```python
from build123d import *

# Parameters (mm, degrees)
SKETCH1_R           = 35
BOSS_EXTRUDE1_DEPTH = 15
CHAMFER2_SIZE       = 7
SKETCH2_R           = 22.041880944
CUT_EXTRUDE1_DEPTH  = 7


with BuildPart() as part:
    # Sketch1 → Boss-Extrude1 (new body)
    with BuildSketch(Plane(origin=(0, 0, 0), x_dir=(1, 0, 0), z_dir=(0, 1, 0))):
        with Locations(Location((1.345738872, 0, 0), (0, 0, 270))):
            Circle(SKETCH1_R)
    extrude(amount=BOSS_EXTRUDE1_DEPTH)

    # Chamfer2
    chamfer2_edges = [part.edges().sort_by_distance(p)[0] for p in [
        (1.345738872, 0, -35),
    ]]
    chamfer(chamfer2_edges, length=CHAMFER2_SIZE)

    # Sketch2 → Cut-Extrude1 (cut)
    with BuildSketch(Plane(origin=(0, 15, 0), x_dir=(1, 0, 0), z_dir=(0, 1, 0))):
        with Locations(Location((0, 0, 0), (0, 0, 270))):
            Circle(SKETCH2_R)
    extrude(amount=-CUT_EXTRUDE1_DEPTH, mode=Mode.SUBTRACT)


solid = part.part
```
Work out the finished part from the listing and answer in its coordinate system (mm). A direction names the side the tool comes from. Coordinates: 2 decimals unless noted, no trailing zeros. Loops run counter-clockwise (first coordinate to the right, second up) from the corner with the lowest first, then second, coordinate; pieces in that order, holes last. Notation, with made-up numbers: M -32,1.5 L 1,1.5 A27 cw 1,33.5 Z; hole C 44,82.5 d10. An arc over 180 degrees is marked long. Use CSV: the item, a comma, the result in double quotes. Start each with the question number.
(1) Find section A-A, the plane z = 0. Give the vertices of the cut face in (x, y).
(2) For faces 4 (the face through (17, 15, 15)), 5 (the face through (6.621, 11.549, 21.024)), determine the directions among +Z, -Z, +X, -X, +Y, -Y from which every point of the face is accessible in a straight line to the end or side of a thin tool.
(3) For a pull along X with two mould halves and no side action, classify faces 1 (the face through (36.048, 10.944, -4.556)), 2 (the face through (2, 0, 0)), 3 (the face through (0, 8, 0)) as +X half, -X half, draft (parallel to the pull), parting line (faces both ways), or undercut.
(4) Find section C-C, the plane y = 4.75. Give the vertices of the cut face in (x, z), then the cut area to 3 significant figures.
(5) Find section B-B, the plane y = 11. Give the vertices of the cut face in (x, z), then the cut area to 3 significant figures.
(6) Given pin 1 Ø4 at (x, y) = (-10, 4.5) entering from -Z; pin 2 Ø10 at (x, z) = (4.5, 0) entering from +Y; pin 3 Ø8 at (x, y) = (15, 11) entering from +Z, each flat-ended and moving along its own axis, determine where each tip first touches the part or whether it passes through.
(7) Consider line 1 (X direction, y = 13.25, z = 0); line 2 (X direction, y = 9.5, z = 4.5); line 3 (Y direction, x = -6, z = -19.5). Determine where each line is inside the solid, lowest interval first.
Recorded:
1,outline,"M -33.65,7 L -26.65,0 L 29.35,0 L 36.35,7 L 36.35,15 L 22.04,15 L 22.04,8 L -22.04,8 L -22.04,15 L -33.65,15 Z"
2,face 4,"+Z, -Z, +X, -X, +Y"
2,face 5,"+Y"
3,face 1,"parting line"
3,face 2,"draft"
3,face 3,"undercut"
4,outline,"C 1.35,0 d65.5"
4,area,"3,370 mm^2"
5,outline,"C 1.35,0 d70; hole C 0,0 d44.08"
5,area,"2,320 mm^2"
6,pin 1,"stops at z = -32.69"
6,pin 2,"stops at y = 8"
6,pin 3,"stops at z = 33.64"
7,line 1,"x = -33.65 to -22.04, 22.04 to 36.35"
7,line 2,"x = -33.36 to -21.58, 21.58 to 36.06"
7,line 3,"y = 0 to 8"
